from build123d import *

# Parameters (mm, degrees)
F0_R     = 40.8737100338
F1_DEPTH = 3
F2_R     = 40.6957539797
F2_R_2   = 38.5419315624
F3_DEPTH = 1.5
F5_DEPTH = 3.5
F6_R     = 2.1975710884
F7_DEPTH = 3


with BuildPart() as f1:
    # F0 (on Top) → F1 (new body)
    with BuildSketch(Plane.XY):
        Circle(F0_R)
    extrude(amount=F1_DEPTH)

    # F2 (on face) → F3 (join)
    with BuildSketch(Plane.XY.offset(3)):
        Circle(F2_R)
        Circle(F2_R_2, mode=Mode.SUBTRACT)
    extrude(amount=F3_DEPTH)

    # F4 (on face) → F5 (join)
    with BuildSketch(Plane.XY.offset(3)):
        with BuildLine():
            add(Edge.make_bspline(
                [(-18.5161922127, 19.791925326), (-12.7151925876, 21.3351674452), (-3.2277425118, 23.859117369), (3.4150540296, 20.4339539585), (6.2694455573, 13.0889481493), (3.9197467048, 8.1734523404), (2.6966251899, 5.6147207506)],
                knots=[0, 0, 0, 0, 0.332446594, 0.5437115441, 0.7624818062, 1, 1, 1, 1], degree=3))
            Line((-18.5161922127, 19.791925326), (-16.20740816, 13.5870669037))
            add(Edge.make_bspline(
                [(-16.20740816, 13.5870669037), (-11.0929458702, 15.6161362843), (-2.752055686, 18.9252319275), (0.6709459709, 12.4764702332), (-0.5376493129, 5.2281596847), (-6.4609189943, 6.24601212), (-9.7139514983, 6.8050120026)],
                knots=[0, 0, 0, 0, 0.3275893752, 0.5342471699, 0.7442106849, 1, 1, 1, 1], degree=3))
            Line((-9.7139514983, 6.8050120026), (-8.7038585916, 2.1874438971))
            add(Edge.make_bspline(
                [(-8.7038585916, 2.1874438971), (-5.0516756353, 1.8971066874), (1.4743799313, 1.3783055249), (0.4320748866, -6.0037109711), (-4.6539335606, -14.2800911607), (-14.7593699815, -14.073892468), (-21.0811542832, -5.254384585), (-24.8474739492, 0)],
                knots=[0, 0, 0, 0, 0.1955278639, 0.3493871254, 0.5461884526, 0.7296333955, 1, 1, 1, 1], degree=3))
            add(Edge.make_bspline(
                [(-24.8474739492, 0), (-21.8108523669, -6.8272496265), (-17.0623369266, -17.5033577248), (-10.2515605655, -19.7180403086), (0.7822052269, -17.4220041674), (7.8494428689, -7.7477839242), (6.0306062721, -2.4276731034), (5.2006347105, 0)],
                knots=[0, 0, 0, 0, 0.2707643094, 0.4234075499, 0.6256267457, 0.8291659872, 1, 1, 1, 1], degree=3))
            add(Edge.make_bspline(
                [(5.2006347105, 0), (7.0558782543, -0.288731548), (10.3259106837, -0.7976466868), (12.5781414282, 2.3991075178), (10.8457845725, 5.4428405295), (11.0488135588, 9.7583543287), (16.3784916805, 9.6098216805), (21.4125144717, 8.4677573473), (22.2506321534, 3.0756632517), (22.7286964655, 0)],
                knots=[0, 0, 0, 0, 0.1522720518, 0.2683930901, 0.393191332, 0.517267269, 0.6610905311, 0.8066852357, 1, 1, 1, 1], degree=3))
            add(Edge.make_bspline(
                [(22.7286964655, 0), (22.3751428346, -2.8940459342), (21.760112666, -7.9284322424), (17.1960973157, -10.7354530989), (12.7814342968, -8.5747040819), (11.6223696105, -4.6521009952), (10.9791178256, -2.475154819)],
                knots=[0, 0, 0, 0, 0.2987774731, 0.5197433814, 0.7334696409, 1, 1, 1, 1], degree=3))
            add(Edge.make_bspline(
                [(10.9791178256, -2.475154819), (10.4143752119, -5.868762178), (9.4170665506, -11.8617117622), (15.7194742185, -13.7352738113), (22.208604559, -12.607886853), (25.7160244182, -4.5211657639), (26.6477559678, 3.6676927283), (24.0516080161, 11.6963261383), (20.3404842083, 14.366500869), (15.9475940403, 16.4684038367), (10.5274427232, 14.8383861124), (9.0509264503, 11.7721150129), (7.1117466969, 6.480918156), (9.3180739858, 4.40547596), (5.5607718644, 3.6452011728), (3.704177681, 4.9218811085), (2.6966251899, 5.6147207506)],
                knots=[0, 0, 0, 0, 0.0927466913, 0.1637862563, 0.2408254215, 0.3302072886, 0.4224188469, 0.511065812, 0.5768972077, 0.6451241214, 0.7155702479, 0.7742736226, 0.8469858668, 0.8895704824, 0.9400711601, 1, 1, 1, 1], degree=3))
        make_face()
        with BuildLine():
            add(Edge.make_bspline(
                [(-11.3643482327, 29.4991154224), (-6.404904251, 28.4573434012), (2.8845705426, 26.5060127748), (9.9821642335, 29.7299226682), (13.2905105129, 31.2326587737)],
                knots=[0, 0, 0, 0, 0.5338777586, 1, 1, 1, 1], degree=3))
            add(Edge.make_bspline(
                [(-11.3643482327, 29.4991154224), (-7.7798241077, 27.8488746747), (-0.6953090811, 24.5873105264), (11.6043928769, 23.9693963536), (14.2279842551, 26.1669657789), (15.2166699991, 26.9951075315)],
                knots=[0, 0, 0, 0, 0.3895762705, 0.76996523, 1, 1, 1, 1], degree=3))
            Line((15.2166699991, 26.9951075315), (13.2905105129, 31.2326587737))
        make_face()
        Polygon((0, 36.3618300318), (-3.4969905391, 33.3261489868), (0, 29.9247764051), (3.2172903236, 33.232509843), align=None)
    extrude(amount=F5_DEPTH)

    # F6 (on face) → F7 (cut)
    with BuildSketch(Plane.XY.offset(3)):
        with Locations((-8.2511557266, 33.6113274097)):
            Circle(F6_R)
    extrude(amount=-F7_DEPTH, mode=Mode.SUBTRACT)


solid = f1.part
Read the model definition and answer for the solid it produces. Units are mm, in the model's axes. A direction names the side the tool comes from. Give positions to 0.01 mm unless a question says otherwise; leave off trailing zeros. Loops run counter-clockwise (first coordinate to the right, second up) from the corner with the lowest first, then second, coordinate; pieces in that order, holes last. Notation, with made-up numbers: (-32.75, -31.5) - (22.25, -31.5) arc R16 ccw to (22.25, -12.5) - close; hole circle Ø9 at (21, 28). An arc over 180 degrees is marked (long way). Answer as CSV lines item,"result". Start each with the question number.
1) Find section A-A (y = -26). Write down the section's boundary in (x, z).
2) Find section B-B (z = 2). Write down the section's boundary in (x, y), then the cut area to 3 significant figures.
3) Straight lines are drawn through the part: L1, parallel to X at y = -6, z = 5.25; L2, parallel to X at y = -8, z = 4; L3, parallel to Y at x = 20.5, z = 3.5. For each, find the intervals that lie inside material, in ascending order. Write a range as from..to.
4) Find section C-C (x = -34). Write down the section's boundary in (y, z), then the cut area to 3 significant figures.
5) Each of these flat-tipped pins is pushed along its axis until it touches: pin 1 Ø1.5 at (y, z) = (-4.5, 1.5) entering from -X; pin 2 Ø24.5 at (x, y) = (14.5, 19.5) entering from +Z; pin 3 Ø3 at (x, y) = (-32, 10) entering from +Z; pin 4 Ø1.5 at (x, z) = (0.5, 2.5) entering from -Y. Where does it stop, or does it pass through?
6) Determine the mould class of faces 1 (the face through (5, 27, 6.5)), 2 (the face through (38.986, 12.277, 1.479)), 3 (the face through (8, -8, 3)) for opening direction Y: released by +Y, released by -Y, zero draft, split by the parting line, or undercut.
7) Which of the six approach directions +Z, -Z, +X, -X, +Y, -Y give full straight-line access (tool end or side, diameter ignored) to faces 4 (the face through (-1, 1, 0)), 5 (the face through (-1.773, 31.649, 4.726))?
Findings below:
1,outline,"(-31.54, 0) - (31.54, 0) - (31.54, 3) - (31.31, 3) - (31.31, 4.5) - (28.45, 4.5) - (28.45, 3) - (-28.45, 3) - (-28.45, 4.5) - (-31.31, 4.5) - (-31.31, 3) - (-31.54, 3) - close"
2,outline,"circle Ø81.75 at (0, 0); hole circle Ø4.4 at (-8.25, 33.61)"
2,area,"5,230 mm^2"
3,L1,"-22.14..-20.4, -0.17..6.51, 10.46..12.16, 21.6..24.82"
3,L2,"-39.9..-37.7, -21.18..-18.73, -1.09..6.24, 10.33..13.28, 20.58..24.04, 37.7..39.9"
3,L3,"-35.16..-32.64, -12.32..-8.1, 7.63..14.12, 32.64..35.16"
4,outline,"(-22.69, 0) - (22.69, 0) - (22.69, 3) - (22.36, 3) - (22.36, 4.5) - (18.15, 4.5) - (18.15, 3) - (-18.15, 3) - (-18.15, 4.5) - (-22.36, 4.5) - (-22.36, 3) - (-22.69, 3) - close"
4,area,"149 mm^2"
5,pin 1,"x = -40.7"
5,pin 2,"z = 6.5"
5,pin 3,"z = 3"
5,pin 4,"y = -40.87"
6,face 1,"zero draft"
6,face 2,"split by the parting line"
6,face 3,"undercut"
7,face 4,"-Z, +X, -X, +Y, -Y"
7,face 5,"+Z"
